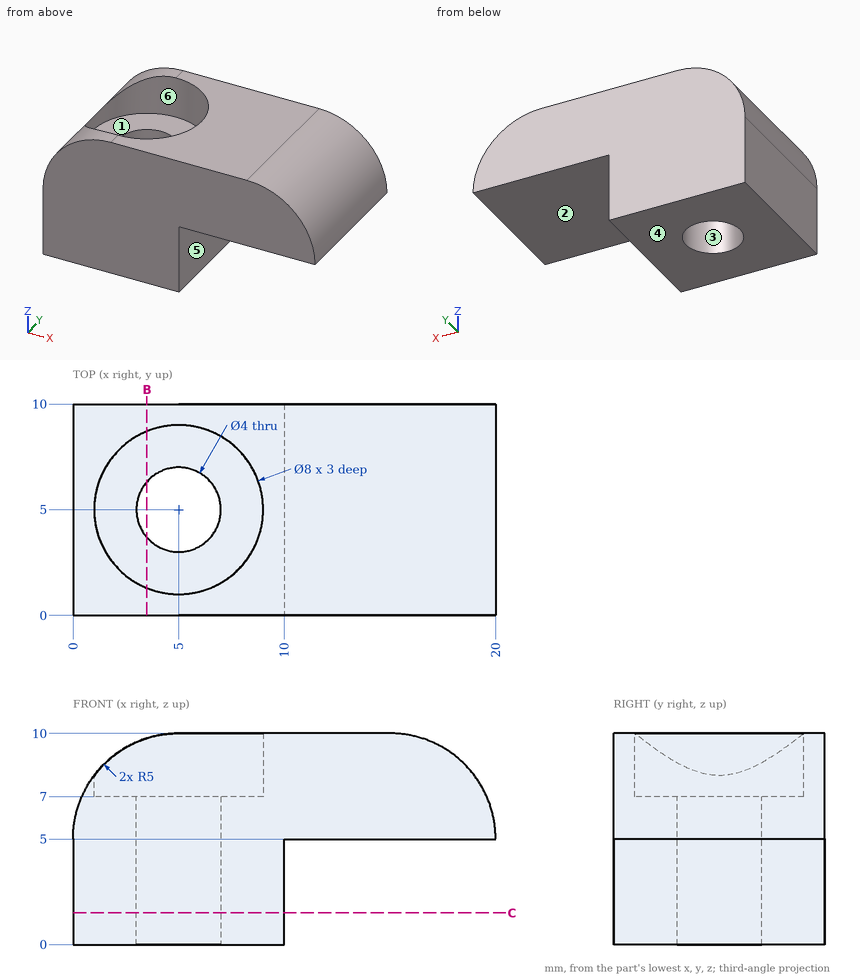
Verification items for this drawing (mm, ordinates from the low corner). A direction names the side the tool comes from. Coordinates: 2 decimals unless noted, no trailing zeros. Write each loop counter-clockwise with the first axis right and the second up, starting at its lowest first coordinate (ties: lowest second). Pieces come first, ordered by that corner, then holes. Notation, with made-up numbers: (83.25, 86.25) -> (126.25, 86.25) arc R26 ccw to (126.25, 124.25) -> close; hole circle Ø1 at (-25, 60.25). An arc over 180 degrees is marked (long way). One line per item, written item: value. Start each with the question number.
Q1. Cross-section at C-C on z = 1.5. Enter the section's corners in (x, y), and give its area (3 significant figures).
Q2. Thickness scan on L1, parallel to Y at x = 5, z = 7.9; L2, parallel to Y at x = 5, z = 2; L3, parallel to Z at x = 12.25, y = 5.5. Record the ranges inside material, lowest first. Write a range as from..to.
Q3. Access from +Z, -Z, +X, -X, +Y, -Y to the whole of each face (thin tool, end or side, straight path). Record for the marked faces 1, 2 and 3.
Q4. Cross-section at B-B on x = 3.5. Enter the section's corners in (y, z), and give its area (3 significant figures).
Q5. Mould release check, pull along X, two halves, no side actions. Record for the marked faces 4, 5 and 6: pulls with the +X half, pulls with the -X half, needs draft (parallel to the pull), parting line crosses it, or undercut.
Q6. Go/stop test with flat-tipped pins: P1, Ø2.5, axis at y = 3.5, z = 3, coming from the +X side; P2, Ø1.5, axis at x = 17.5, y = 2, coming from the +Z side; P3, Ø2, axis at y = 7.5, z = 8, coming from the -X side. Record where each tip stops, or that it passes through.
Checked values:
1. outline: (0, 0) -> (10, 0) -> (10, 10) -> (0, 10) -> close; hole circle Ø4 at (5, 5)
1. area: 87.4 mm²
2. L1: y = 0..1, 9..10
2. L2: y = 0..3, 7..10
2. L3: z = 5..10
3. face 1: +Z
3. face 2: -Z, +X, +Y, -Y
3. face 3: +Z, -Z
4. outline: (0, 0) -> (3.68, 0) -> (3.68, 7) -> (1.29, 7) -> (1.29, 9.77) -> (0, 9.77) -> close; (6.32, 0) -> (10, 0) -> (10, 9.77) -> (8.71, 9.77) -> (8.71, 7) -> (6.32, 7) -> close
4. area: 58.6 mm²
5. face 4: needs draft
5. face 5: pulls with the +X half
5. face 6: undercut
6. P1: stops at x = 10
6. P2: stops at z = 9.68
6. P3: stops at x = 0.42
